The listing builds one solid part. Answer for the finished solid, in the listing's coordinates (mm). A direction names the side the tool comes from. Round coordinates to 2 decimals unless told otherwise and drop trailing zeros. Write each loop counter-clockwise with the first axis right and the second up, starting at its lowest first coordinate (ties: lowest second). Pieces come first, ordered by that corner, then holes.
from build123d import *

# Parameters (mm, degrees)
SKETCH1_W           = 33
SKETCH1_H           = 60
SKETCH1_R           = 1
SKETCH1_W_2         = 23
SKETCH1_H_2         = 12.5
SKETCH1_W_3         = 6
SKETCH1_H_3         = 6
BOSS_EXTRUDE1_DEPTH = 5
SKETCH2_R           = 0.85
CUT_EXTRUDE1_DEPTH  = 3
CUT_EXTRUDE2_START  = -3
SKETCH3_R           = 0.85
CUT_EXTRUDE2_DEPTH  = 3
FILLET1_R           = 3


with BuildPart() as part:
    # Sketch1 → Boss-Extrude1 (new body)
    with BuildSketch(Plane.XY):
        Rectangle(SKETCH1_W, SKETCH1_H)
        with Locations((-14.65, 21.75)):
            Circle(SKETCH1_R, mode=Mode.SUBTRACT)
        with Locations(Location((14.65, 21.75, 0), (0, 0, 180))):
            Circle(SKETCH1_R, mode=Mode.SUBTRACT)
        with Locations((14.65, -21.75)):
            Circle(SKETCH1_R, mode=Mode.SUBTRACT)
        with Locations(Location((-14.65, -21.75, 0), (0, 0, 180))):
            Circle(SKETCH1_R, mode=Mode.SUBTRACT)
        with Locations((0, 21.75)):
            Rectangle(SKETCH1_W_2, SKETCH1_H_2, mode=Mode.SUBTRACT)
        with Locations((0, -21.75)):
            Rectangle(SKETCH1_W_2, SKETCH1_H_2, mode=Mode.SUBTRACT)
        with Locations((11.5, 0)):
            Rectangle(SKETCH1_W_3, SKETCH1_H_3, mode=Mode.SUBTRACT)
        with Locations((-11.5, 0)):
            Rectangle(SKETCH1_W_3, SKETCH1_H_3, mode=Mode.SUBTRACT)
    extrude(amount=BOSS_EXTRUDE1_DEPTH)

    # Sketch2 → Cut-Extrude1 (cut)
    with BuildSketch(Plane(origin=(16.5, 0, 0), x_dir=(0, 0, -1), z_dir=(1, 0, 0))):
        with Locations((-2.5, 0)):
            Circle(SKETCH2_R)
    extrude(amount=-CUT_EXTRUDE1_DEPTH, mode=Mode.SUBTRACT)

    # Sketch3 → Cut-Extrude2 (cut)
    with BuildSketch(Plane.ZY.offset(16.5).offset(CUT_EXTRUDE2_START)):
        with Locations(Location((2.5, 0, 0), (0, 0, 180))):
            Circle(SKETCH3_R)
    extrude(amount=CUT_EXTRUDE2_DEPTH, mode=Mode.SUBTRACT)

    # Fillet1
    fillet1_edges = [part.edges().sort_by_distance(p)[0] for p in [
        (16.5, -30, 2.5),
        (-16.5, -30, 2.5),
        (-16.5, 30, 2.5),
        (16.5, 30, 2.5),
    ]]
    fillet(fillet1_edges, radius=FILLET1_R)


solid = part.part
1. Section D-D on y = -21.75 is taken. Determine the outline of the cut face in (x, z).
Geometry says:
outline: (-16.5, 0) - (-15.65, 0) - (-15.65, 5) - (-16.5, 5) - close; (-13.65, 0) - (-11.5, 0) - (-11.5, 5) - (-13.65, 5) - close; (11.5, 0) - (13.65, 0) - (13.65, 5) - (11.5, 5) - close; (15.65, 0) - (16.5, 0) - (16.5, 5) - (15.65, 5) - close
2. Section A-A on x = 5 is taken. Determine the outline of the cut face in (y, z), plus the area to 3 significant figures.
Geometry says:
outline: (-30, 0) - (-28, 0) - (-28, 5) - (-30, 5) - close; (-15.5, 0) - (15.5, 0) - (15.5, 5) - (-15.5, 5) - close; (28, 0) - (30, 0) - (30, 5) - (28, 5) - close
area: 175 mm2
3. Section C-C on x = 9.5 is taken. Determine the outline of the cut face in (y, z), plus the area to 3 significant figures.
Geometry says:
outline: (-30, 0) - (-28, 0) - (-28, 5) - (-30, 5) - close; (-15.5, 0) - (-3, 0) - (-3, 5) - (-15.5, 5) - close; (3, 0) - (15.5, 0) - (15.5, 5) - (3, 5) - close; (28, 0) - (30, 0) - (30, 5) - (28, 5) - close
area: 145 mm2
4. Straight lines are drawn through the part: line 1 along Y through (x, z) = (2, 3.75); line 2 along X through (y, z) = (-2, 4); line 3 along Y through (x, z) = (14.65, 2.5). For each, find the intervals that lie inside material, in ascending order.
Geometry says:
line 1: y = -30 to -28, -15.5 to 15.5, 28 to 30
line 2: x = -16.5 to -14.5, -8.5 to 8.5, 14.5 to 16.5
line 3: y = -29.77 to -22.75, -20.75 to -0.85, 0.85 to 20.75, 22.75 to 29.77
5. Given pin 1 (2.5 mm diameter, centred on y = 0, z = 2.5, fed in from -X); pin 2 (1.6 mm diameter, centred on x = -14.65, y = -21.75, fed in from -Z), each flat-ended and moving along its own axis, determine where each tip first touches the part or whether it passes through.
Geometry says:
pin 1: stops at x = -16.5
pin 2: passes through
6. Section B-B on y = 0 is taken. Determine the outline of the cut face in (x, z), plus the area to 3 significant figures.
Geometry says:
outline: (-16.5, 0) - (-14.5, 0) - (-14.5, 1.65) - (-16.5, 1.65) - close; (-16.5, 3.35) - (-14.5, 3.35) - (-14.5, 5) - (-16.5, 5) - close; (-8.5, 0) - (8.5, 0) - (8.5, 5) - (-8.5, 5) - close; (14.5, 0) - (16.5, 0) - (16.5, 1.65) - (14.5, 1.65) - close; (14.5, 3.35) - (16.5, 3.35) - (16.5, 5) - (14.5, 5) - close
area: 98.2 mm2
7. For a pull along X with two mould halves and no side action, classify faces 4 (the face through (-14.433, -20.774, 2.465)), 5 (the face through (15.6, -29.14, 2.54)), 6 (the face through (-15.64, 29.1, 2.54)) as released by +X, released by -X, zero draft, split by the parting line, or undercut.
Geometry says:
face 4: undercut
face 5: released by +X
face 6: released by -X
8. A tool of negligible diameter and unlimited length cuts with its end or side. For faces 1 (the face through (-11.5, 22, 2)), 2 (the face through (-15.486, 0.326, 1.715)), 3 (the face through (16.5, 0, 1)), from which of +Z, -Z, +X, -X, +Y, -Y can it reach the whole face along a straight path? Write none if from no direction.
Geometry says:
face 1: +Z, -Z
face 2: -X
face 3: +Z, -Z, +X, +Y, -Y
